```python
from build123d import *

# Parameters (mm, degrees)
F0_W      = 5
F0_H      = 70
F1_DEPTH  = 50
F2_R      = 23.75
F3_DEPTH  = 40
F4_R      = 16.352072
F5_DEPTH  = 10
F6_R      = 3.75
F7_DEPTH  = 30
F8_R      = 3.75
F9_DEPTH  = 5
F10_R     = 15
F11_DEPTH = 15


with BuildPart() as f1:
    # F0 (on Front) → F1 (new body)
    with BuildSketch(Plane.XZ):
        with Locations((0, 35.574075)):
            Rectangle(F0_W, F0_H)
    extrude(amount=-F1_DEPTH)

    # F2 (on face) → F3 (join)
    with BuildSketch(Plane(origin=(-2.5, 0, 0), x_dir=(0, -1, 0), z_dir=(-1, 0, 0))):
        with Locations((-24.496011, 45.235008)):
            Circle(F2_R)
    extrude(amount=F3_DEPTH)

    # F4 (on face) → F5 (join)
    with BuildSketch(Plane(origin=(-42.5, 0, 0), x_dir=(0, -1, 0), z_dir=(-1, 0, 0))):
        with Locations((-24.496011, 45.235008)):
            Circle(F4_R)
    extrude(amount=F5_DEPTH)

    # F6 (on face) → F7 (join)
    with BuildSketch(Plane(origin=(-52.5, 0, 0), x_dir=(0, -1, 0), z_dir=(-1, 0, 0))):
        with Locations((-24.496011, 45.235008)):
            Circle(F6_R)
    extrude(amount=F7_DEPTH)

    # F8 (on face) → F9 (join)
    with BuildSketch(Plane.YZ.offset(2.5)):
        with Locations((25.3156, 45.039263)):
            Circle(F8_R)
    extrude(amount=F9_DEPTH)

    # F10 (on face) → F11 (join)
    with BuildSketch(Plane.YZ.offset(7.5)):
        with Locations((25.3156, 45.039263)):
            Circle(F10_R)
    extrude(amount=F11_DEPTH)


solid = f1.part
```
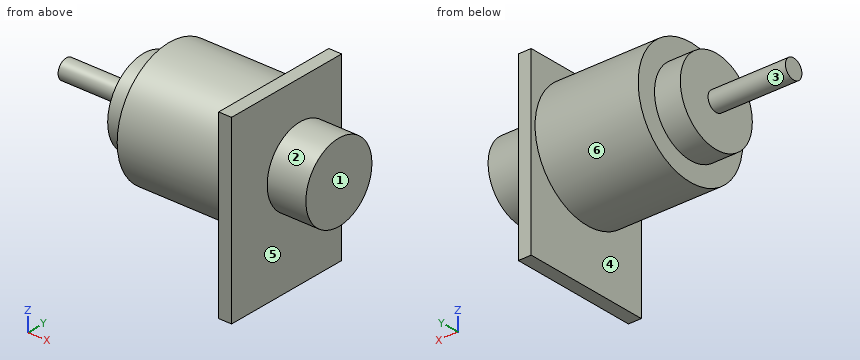
CAD build for the part. Positions are in the model's coordinates, mm. Face numbers are marked on the shaded views. A direction names the side the tool comes from. Coordinates: 2 decimals unless noted, no trailing zeros. Write each loop counter-clockwise with the first axis right and the second up, starting at its lowest first coordinate (ties: lowest second). Pieces come first, ordered by that corner, then holes. Notation, with made-up numbers: (56, 63.5) -> (78, 63.5) arc R32 ccw to (78, 98.5) -> close; hole circle Ø2 at (11, 7). An arc over 180 degrees is marked (long way). Use CSV: the item, a comma, the result in double quotes. Start each with the question number.
Item 1: Two-plate mould, pull along X, no slides. Class the marked faces 4, 5 and 6: +X half, -X half, draft (parallel to the pull), parting line (faces both ways), or undercut.
Item 2: Band-saw the part on B-B, the plane y = 31.5. Write the cut outline in (x, z), plus the area to 3 significant figures.
Item 3: Tool access for the marked faces 1, 2 and 3: list every direction of +Z, -Z, +X, -X, +Y, -Y with a clear straight run to the whole face (end or side of a thin tool).
Item 4: Band-saw the part on C-C, the plane y = 44. Write the cut outline in (x, z).
Item 5: Drop flat-ended pins along their axis: P1, Ø8, axis at y = 37.5, z = 52, coming from the -X side; P2, Ø1.5, axis at x = -39, y = 23, coming from the -Z side; P3, Ø8, axis at x = -17.5, y = 40.5, coming from the +Z side; P4, Ø1, axis at x = -53.5, y = 36.5, coming from the +Z side. Give the stop position or say it passes through.
Item 6: Wall check: probe 1 along X at (y, z) = (24.5, 58); probe 2 along X at (y, z) = (13, 16.5); probe 3 along X at (y, z) = (42, 42). Give the ranges that are in metal, low to high.
Item 7: Band-saw the part on A-A, the plane z = 36.5. Write the cut outline in (x, y).
Item 8: Band-saw the part on D-D, the plane z = 12.5. Write the cut outline in (x, y).
Response values:
1,face 4,"-X half"
1,face 5,"undercut"
1,face 6,"draft"
2,outline,"(-52.5, 30.46) -> (-42.5, 30.46) -> (-42.5, 22.54) -> (-2.5, 22.54) -> (-2.5, 0.57) -> (2.5, 0.57) -> (2.5, 70.57) -> (-2.5, 70.57) -> (-2.5, 67.93) -> (-42.5, 67.93) -> (-42.5, 60.01) -> (-52.5, 60.01) -> close; (7.5, 31.37) -> (22.5, 31.37) -> (22.5, 58.71) -> (7.5, 58.71) -> close"
2,area,"2,870 mm2"
3,face 1,"+Z, -Z, +X, +Y, -Y"
3,face 2,"+X"
3,face 3,"-X"
4,outline,"(-42.5, 31.68) -> (-2.5, 31.68) -> (-2.5, 0.57) -> (2.5, 0.57) -> (2.5, 70.57) -> (-2.5, 70.57) -> (-2.5, 58.79) -> (-42.5, 58.79) -> close"
5,P1,"stops at x = -52.5"
5,P2,"stops at z = 21.5"
5,P3,"stops at z = 65.73"
5,P4,"passes through"
6,probe 1,"x = -52.5 to 2.5, 7.5 to 22.5"
6,probe 2,"x = -2.5 to 2.5"
6,probe 3,"x = -42.5 to 2.5"
7,outline,"(-52.5, 10.67) -> (-42.5, 10.67) -> (-42.5, 2.41) -> (-2.5, 2.41) -> (-2.5, 0) -> (2.5, 0) -> (2.5, 50) -> (-2.5, 50) -> (-2.5, 46.58) -> (-42.5, 46.58) -> (-42.5, 38.32) -> (-52.5, 38.32) -> close; (7.5, 12.98) -> (22.5, 12.98) -> (22.5, 37.65) -> (7.5, 37.65) -> close"
8,outline,"(-2.5, 0) -> (2.5, 0) -> (2.5, 50) -> (-2.5, 50) -> close"
